The listing builds one solid part. Answer for the finished solid, in the listing's coordinates (mm). Face numbers are marked on the shaded views. Coordinates: 2 decimals unless noted, no trailing zeros. Loops run counter-clockwise (first coordinate to the right, second up) from the corner with the lowest first, then second, coordinate; pieces in that order, holes last. Notation, with made-up numbers: (-27.5, 4) -> (-6.5, 4) arc R37 cw to (-6.5, 41) -> close; hole circle Ø9 at (24, 48.25). An arc over 180 degrees is marked (long way). Answer in a Markdown table with one row per item.
```python
from build123d import *

# Parameters (mm, degrees)
F0_R     = 15.875
F1_DEPTH = 38.1


with BuildPart() as f1:
    # F0 (on Front) → F1 (new body)
    with BuildSketch(Plane.XZ):
        Polygon((24.201399, -89.930544), (92.873329, -16.472389), (105.252468, 83.320855), (56.610405, 171.33156), (-34.473246, 213.942629), (-133.207625, 194.878081), (-201.879555, 121.419927), (-214.258694, 21.626683), (-165.616631, -66.384023), (-74.532981, -108.995092), align=None)
        with Locations((-147.017439, -46.488524)):
            Circle(F0_R, mode=Mode.SUBTRACT)
        with Locations((-71.180199, -81.966965)):
            Circle(F0_R, mode=Mode.SUBTRACT)
        with Locations((-187.517351, 26.790149)):
            Circle(F0_R, mode=Mode.SUBTRACT)
        with Locations((11.027121, -66.093614)):
            Circle(F0_R, mode=Mode.SUBTRACT)
        with Locations((68.204119, -4.931554)):
            Circle(F0_R, mode=Mode.SUBTRACT)
        with Locations((-177.210345, 109.879091)):
            Circle(F0_R, mode=Mode.SUBTRACT)
        with Locations((-120.033347, 171.041152)):
            Circle(F0_R, mode=Mode.SUBTRACT)
        with Locations((78.511125, 78.157389)):
            Circle(F0_R, mode=Mode.SUBTRACT)
        with Locations((-37.826027, 186.914502)):
            Circle(F0_R, mode=Mode.SUBTRACT)
        with Locations((38.011213, 151.436061)):
            Circle(F0_R, mode=Mode.SUBTRACT)
    extrude(amount=-F1_DEPTH)


solid = f1.part
```
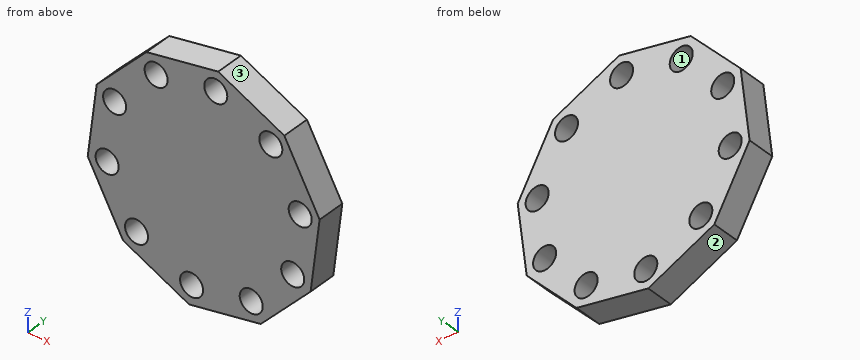
Item 1: Determine the mould class of the marked faces 1, 2 and 3 for opening direction X: +X half, -X half, draft (parallel to the pull), parting line (faces both ways), or undercut.
Findings below:
| item | result |
|---|---|
| face 1 | undercut |
| face 2 | -X half |
| face 3 | +X half |
Item 2: Flat-ended cylindrical pins translate along their axes: pin 1 Ø1.5 at (x, y) = (-174.5, 25) entering from +Z; pin 2 Ø10 at (x, y) = (-43, 29.5) entering from +Z; pin 3 Ø10 at (x, y) = (-96, 13.5) entering from -Z; pin 4 Ø5 at (x, z) = (-167, 116.5) entering from +Y. Find the tip coordinate at first contact, or state that the pin passes through.
Findings below:
| item | result |
|---|---|
| pin 1 | stops at z = 151.51 |
| pin 2 | stops at z = 213.26 |
| pin 3 | stops at z = -101.29 |
| pin 4 | passes through |
Item 3: A cutting plane is placed at C-C, the plane y = 32.5. Count the separate pieces of the cut face and the enclosed holes in it, plus the area to 3 significant figures.
Findings below:
| item | result |
|---|---|
| separate pieces | 1 |
| enclosed holes | 10 |
| area | 69,900 mm2 |
Item 4: A cutting plane is placed at A-A, the plane z = 73. Determine the outline of the cut face in (x, y).
Findings below:
| item | result |
|---|---|
| outline | (-207.89, 0) -> (63.5, 0) -> (63.5, 38.1) -> (-207.89, 38.1) -> close; (93.53, 0) -> (103.97, 0) -> (103.97, 38.1) -> (93.53, 38.1) -> close |
Item 5: Find the intervals of material crossed by probe 1 along X at (y, z) = (18, 165); probe 2 along X at (y, z) = (13, 161.5); probe 3 along Z at (x, y) = (-191, 34), in increasing order.
Findings below:
| item | result |
|---|---|
| probe 1 | x = -161.14 to -134.71, -105.35 to 29.76, 46.26 to 60.11 |
| probe 2 | x = -164.41 to -132.72, -107.35 to 25.73, 50.29 to 62.04 |
| probe 3 | z = -20.46 to 11.3, 42.28 to 102.01, 117.74 to 133.06 |
Item 6: A cutting plane is placed at B-B, the plane x = -26.5. Determine the outline of the cut face in (y, z), plus the area to 3 significant figures.
Findings below:
| item | result |
|---|---|
| outline | (0, -99.72) -> (38.1, -99.72) -> (38.1, 175.79) -> (0, 175.79) -> close; (0, 198.04) -> (38.1, 198.04) -> (38.1, 210.21) -> (0, 210.21) -> close |
| area | 11,000 mm2 |
